Could you check a few things on this drawing? It's one solid part, dimensions in mm from its lowest x, y, z. A direction names the side the tool comes from. Coordinates: 2 decimals unless noted, no trailing zeros. Loops run counter-clockwise (first coordinate to the right, second up) from the corner with the lowest first, then second, coordinate; pieces in that order, holes last.
1) For the marked faces 1 and 2, which set-ups out of +Z, -Z, +X, -X, +Y, -Y let a thin tool reach every point of the face, with its end or its side?
2) If I drill on line 1 along X through (y, z) = (155, 7.35); line 2 along X through (y, z) = (155, 3); line 3 along Y through (x, z) = (80.5, 7), over which ranges is the centre line in solid material (lowest first)?
3) Imagine slicing it at B-B on x = 126.5. Please give me the cut outline in (y, z).
4) Will these pins go through, and if not, where does the flat tip stop? P1, Ø3, axis at x = 2.5, y = 155, coming from the +Z side; P2, Ø4, axis at x = 227.5, y = 3, coming from the -Z side; P3, Ø3, axis at y = 123.5, z = 3, coming from the +X side.
5) Imagine slicing it at A-A on y = 98. Please give me the cut outline in (x, z), plus the area to 3 significant figures.
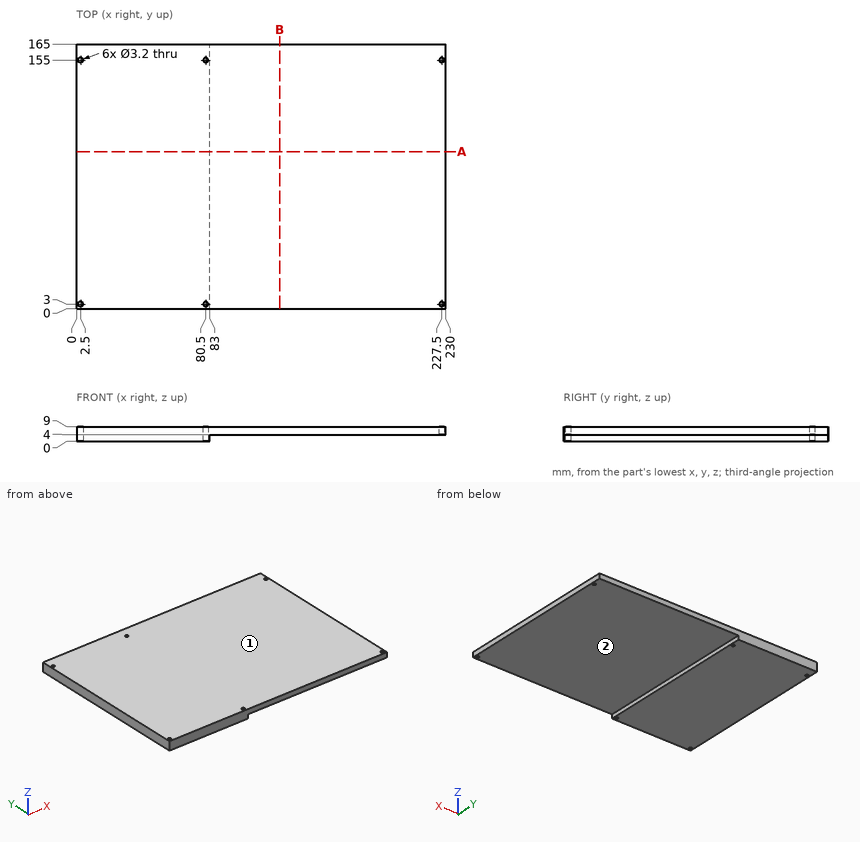
Filled in:
1. face 1: +Z, +X, -X, +Y, -Y
1. face 2: -Z, +X, +Y, -Y
2. line 1: x = 0 to 0.9, 4.1 to 78.9, 82.1 to 225.9, 229.1 to 230
2. line 2: x = 0 to 0.9, 4.1 to 78.9, 82.1 to 83
2. line 3: y = 0 to 1.4, 4.6 to 153.4, 156.6 to 165
3. outline: (0, 4) - (165, 4) - (165, 9) - (0, 9) - close
4. P1: passes through
4. P2: stops at z = 4
4. P3: stops at x = 230
5. outline: (0, 0) - (83, 0) - (83, 4) - (230, 4) - (230, 9) - (0, 9) - close
5. area: 1,480 mm2
